CAD build for the part. Positions are in the model's coordinates, mm. Round coordinates to 2 decimals unless told otherwise and drop trailing zeros. Loops run counter-clockwise (first coordinate to the right, second up) from the corner with the lowest first, then second, coordinate; pieces in that order, holes last. Notation, with made-up numbers: M 39.25,51.5 L 77.25,51.5 A14 ccw 77.25,75.5 Z; hole C 47,10 d8. An arc over 180 degrees is marked long. Put each result on its own line as item: value. Start each with the question number.
from build123d import *

# Parameters (mm, degrees)
BOSS_EXTRUDE1_DEPTH = 6.35
BOSS_EXTRUDE1_DRAFT = -5
CUT_EXTRUDE3_DEPTH  = 15.892070037
CIRPATTERN3_COUNT   = 12
BOSS_EXTRUDE3_DEPTH = 6.35
BOSS_EXTRUDE3_DRAFT = -5
FILLET2_R           = 0.381
BOSS_EXTRUDE4_REACH = 16.734
SKETCH8_R           = 1.1811
SKETCH9_R           = 1.1811
CUT_EXTRUDE4_DEPTH  = 15.73364215
CIRPATTERN4_COUNT   = 4


with BuildPart() as part:
    # Sketch1 → Boss-Extrude1 (with draft: the straight prism first)
    with BuildSketch(Plane(origin=(0, 0, 0), x_dir=(1, 0, 0), z_dir=(0, 1, 0))):
        with BuildLine():
            Line((-6.35, -9.525), (6.35, -9.525))
            ThreePointArc((6.35, -9.525), (8.59506403, -8.59506403), (9.525, -6.35))
            Line((9.525, -6.35), (9.525, 6.35))
            ThreePointArc((9.525, 6.35), (8.59506403, 8.59506403), (6.35, 9.525))
            Line((6.35, 9.525), (-6.35, 9.525))
            ThreePointArc((-6.35, 9.525), (-8.59506403, 8.59506403), (-9.525, 6.35))
            Line((-9.525, 6.35), (-9.525, -6.35))
            ThreePointArc((-9.525, -6.35), (-8.59506403, -8.59506403), (-6.35, -9.525))
        make_face()
    extrude(amount=-BOSS_EXTRUDE1_DEPTH)
    # Boss-Extrude1: the draft: its side faces are tilted about the plane it starts from
    boss_extrude1_sides = [part.faces().sort_by_distance(p)[0] for p in [
        (-8.59506403, -3.175, 8.59506403),
        (0, -3.175, 9.525),
        (8.59506403, -3.175, 8.59506403),
        (9.525, -3.175, 0),
        (8.59506403, -3.175, -8.59506403),
        (0, -3.175, -9.525),
        (-8.59506403, -3.175, -8.59506403),
        (-9.525, -3.175, 0),
    ]]
    draft(boss_extrude1_sides, Plane(origin=(0, 0, 0), x_dir=(1, 0, 0), z_dir=(0, 1, 0)), BOSS_EXTRUDE1_DRAFT)

    # Sketch6 → Cut-Extrude3 (cut, through all)
    with BuildSketch(Plane(origin=(0, 0, 0), x_dir=(0.9659258262890681, 0, 0.25881904510252135), z_dir=(-0.25881904510252135, 0, 0.9659258262890681))):
        Polygon((0, -2.159), (-7.366, -9.525), (7.366, -9.525), align=None)
    cut_extrude3 = extrude(amount=-CUT_EXTRUDE3_DEPTH, mode=Mode.SUBTRACT)

    # CirPattern3: Cut-Extrude3 ×12 about axis
    cirpattern3_axis = Axis((0, 0, 0), (0, 1, 0))
    for i in range(1, CIRPATTERN3_COUNT):
        add(cut_extrude3.rotate(cirpattern3_axis, i * 360 / CIRPATTERN3_COUNT), mode=Mode.SUBTRACT)


with BuildPart() as boss_extrude3_tool:
    # Sketch7 → Boss-Extrude3 (with draft: the straight prism first)
    with BuildSketch(Plane(origin=(0, 0, 0), x_dir=(1, 0, 0), z_dir=(0, 1, 0))):
        with BuildLine():
            Line((-6.35, -9.525), (6.35, -9.525))
            ThreePointArc((6.35, -9.525), (8.59506403, -8.59506403), (9.525, -6.35))
            Line((9.525, -6.35), (9.525, 6.35))
            ThreePointArc((9.525, 6.35), (8.59506403, 8.59506403), (6.35, 9.525))
            Line((6.35, 9.525), (-6.35, 9.525))
            ThreePointArc((-6.35, 9.525), (-8.59506403, 8.59506403), (-9.525, 6.35))
            Line((-9.525, 6.35), (-9.525, -6.35))
            ThreePointArc((-9.525, -6.35), (-8.59506403, -8.59506403), (-6.35, -9.525))
        make_face()
        with BuildLine():
            Line((-6.35, -7.493), (6.35, -7.493))
            ThreePointArc((6.35, -7.493), (7.158223051, -7.158223051), (7.493, -6.35))
            Line((7.493, -6.35), (7.493, 6.35))
            ThreePointArc((7.493, 6.35), (7.158223051, 7.158223051), (6.35, 7.493))
            Line((6.35, 7.493), (-6.35, 7.493))
            ThreePointArc((-6.35, 7.493), (-7.158223051, 7.158223051), (-7.493, 6.35))
            Line((-7.493, 6.35), (-7.493, -6.35))
            ThreePointArc((-7.493, -6.35), (-7.158223051, -7.158223051), (-6.35, -7.493))
        make_face(mode=Mode.SUBTRACT)
    extrude(amount=-BOSS_EXTRUDE3_DEPTH)
    # Boss-Extrude3: the draft: its side faces are tilted about the plane it starts from
    boss_extrude3_sides = [boss_extrude3_tool.faces().sort_by_distance(p)[0] for p in [
        (0, -3.175, 9.525),
        (8.59506403, -3.175, 8.59506403),
        (9.525, -3.175, 0),
        (8.59506403, -3.175, -8.59506403),
        (0, -3.175, -9.525),
        (-8.59506403, -3.175, -8.59506403),
        (-9.525, -3.175, 0),
        (-8.59506403, -3.175, 8.59506403),
        (-7.158223051, -3.175, 7.158223051),
        (-7.493, -3.175, 0),
        (-7.158223051, -3.175, -7.158223051),
        (0, -3.175, -7.493),
        (7.158223051, -3.175, -7.158223051),
        (7.493, -3.175, 0),
        (7.158223051, -3.175, 7.158223051),
        (0, -3.175, 7.493),
    ]]
    draft(boss_extrude3_sides, Plane(origin=(0, 0, 0), x_dir=(1, 0, 0), z_dir=(0, 1, 0)), BOSS_EXTRUDE3_DRAFT)


with BuildPart() as part_1:
    add(part.part)

    # Boss-Extrude3: add boss_extrude3_tool
    add(boss_extrude3_tool.part)

    # Fillet2
    fillet2_edges = [part_1.edges().sort_by_distance(p)[0] for p in [
        (8.202228727, -6.35, -8.202228727),
        (8.202228727, -6.35, 8.202228727),
        (-8.202228727, -6.35, 8.202228727),
        (-8.202228727, -6.35, -8.202228727),
        (-8.969446987, -6.35, 0),
        (0, -6.35, -8.969446987),
        (0, -6.35, 8.969446987),
        (8.969446987, -6.35, 0),
        (-8.048553013, -6.35, 0),
        (-7.551058354, -6.35, 7.551058354),
        (0, -6.35, 8.048553013),
        (7.551058354, -6.35, 7.551058354),
        (8.048553013, -6.35, 0),
        (7.551058354, -6.35, -7.551058354),
        (0, -6.35, -8.048553013),
        (-7.551058354, -6.35, -7.551058354),
    ]]
    fillet(fillet2_edges, radius=FILLET2_R)

    # Sketch8 → Boss-Extrude4 (add, up to next)
    with BuildSketch(Plane(origin=(0, -5.969, 0), x_dir=(-1, 0, 0), z_dir=(0, -1, 0)), mode=Mode.PRIVATE) as boss_extrude4_sk1:
        with Locations((0, 7.493)):
            Circle(SKETCH8_R)
    boss_extrude4_tool1 = extrude(boss_extrude4_sk1.sketch, amount=-BOSS_EXTRUDE4_REACH, mode=Mode.PRIVATE) - part_1.part
    boss_extrude4 = boss_extrude4_tool1.solids().sort_by_distance((0, -5.969, -7.493))[0]
    add(boss_extrude4)

    # Sketch9 → Cut-Extrude4 (cut, through all)
    with BuildSketch(Plane.XZ.offset(5.969)):
        with Locations((0, -7.493)):
            Circle(SKETCH9_R)
    cut_extrude4 = extrude(amount=CUT_EXTRUDE4_DEPTH, mode=Mode.SUBTRACT)

    # CirPattern4: Boss-Extrude4, Cut-Extrude4 ×4 about axis
    cirpattern4_axis = Axis((0, 0, 0), (0, 1, 0))
    add([boss_extrude4.rotate(cirpattern4_axis, i * 360 / CIRPATTERN4_COUNT) for i in range(1, CIRPATTERN4_COUNT)])
    add([cut_extrude4.rotate(cirpattern4_axis, i * 360 / CIRPATTERN4_COUNT) for i in range(1, CIRPATTERN4_COUNT)], mode=Mode.SUBTRACT)


solid = part_1.part
(1) Cut at B-B on y = -5.5. List the corners of the cut face in (x, z), and give its area (3 significant figures).
(2) Drill centre lines: line 1 along X through (y, z) = (-3.5, -7); line 2 along Z through (x, y) = (-4.25, -2.75); line 3 along Z through (x, y) = (-7.5, -4). Where is each one in solid material? Low to high.
(3) Cut at A-A on z = 5. List the corners of the cut face in (x, y) (3 decimals), and give its area (3 significant figures).
(4) Cut at D-D on y = -1.5. List the corners of the cut face in (x, z), and give its area (3 significant figures).
(5) Cut at C-C on x = -5.25. List the corners of the cut face in (y, z) (3 decimals).
(6) Mould opens along Z. For faces 1 (the cylindrical face through (0.034, -4.45, -6.312)), 2 (the flat face through (-4.96, -2.83, -2.024)) say: +Z half, -Z half, draft (parallel to the pull), parting line (faces both ways), or undercut.
(7) Flat gauge pins, fed straight in: pin 1 Ø1.5 at (x, z) = (1, -2) entering from +Y; pin 2 Ø1 at (x, y) = (2, -4) entering from +Z; pin 3 Ø1.5 at (x, z) = (-4, -7) entering from -Y; pin 4 Ø1.2 at (x, z) = (0, 8) entering from -Y. Where does each tip first touch, or does it go through?
Taken from the geometry:
1. outline: M -9.04,-6.35 A2.69 ccw -6.35,-9.04 L 6.35,-9.04 A2.69 ccw 9.04,-6.35 L 9.04,6.35 A2.69 ccw 6.35,9.04 L -6.35,9.04 A2.69 ccw -9.04,6.35 Z; hole M -7.97,-6.35 A1.62 ccw -6.35,-7.97 L -1.08,-7.97 A1.18 cw long 1.08,-7.97 L 6.35,-7.97 A1.62 ccw 7.97,-6.35 L 7.97,-1.08 A1.18 cw long 7.97,1.08 L 7.97,6.35 A1.62 ccw 6.35,7.97 L 1.08,7.97 A1.18 cw long -1.08,7.97 L -6.35,7.97 A1.62 ccw -7.97,6.35 L -7.97,1.08 A1.18 cw long -7.97,-1.08 Z
1. area: 82.0 mm2
2. line 1: -9.14 to -7.65, -5.1 to -3.26, -1.07 to 1.07, 3.26 to 5.1, 7.65 to 9.14
2. line 2: -9.28 to -5.09, -3.41 to -1.75, -0.53 to 0.53, 1.75 to 3.41, 5.09 to 9.28
2. line 3: -8.93 to -7.3, -4.9 to -3.92, -1.18 to 1.18, 3.92 to 4.9, 7.3 to 8.93
3. outline: M -9.525,0 L -9,-6.002 A0.381 ccw -8.62,-6.35 L -8.398,-6.35 A0.381 ccw -8.018,-6.002 L -7.859,-4.18 L -5,-2.159 L -2.887,-3.653 L -1.34,-2.159 L 0,-3.453 L 1.34,-2.159 L 2.887,-3.653 L 5,-2.159 L 7.859,-4.18 L 8.018,-6.002 A0.381 ccw 8.398,-6.35 L 8.62,-6.35 A0.381 ccw 9,-6.002 L 9.525,0 Z
3. area: 64.0 mm2
4. outline: M -9.39,-6.35 A3.04 ccw -6.35,-9.39 L 6.35,-9.39 A3.04 ccw 9.39,-6.35 L 9.39,6.35 A3.04 ccw 6.35,9.39 L -6.35,9.39 A3.04 ccw -9.39,6.35 Z
4. area: 345 mm2
5. outline: M -6.35,-8.62 A0.381 ccw -6.002,-9 L 0,-9.525 L 0,9.525 L -6.002,9 A0.381 ccw -6.35,8.62 L -6.35,8.398 A0.381 ccw -6.002,8.018 L -3.992,7.842 L -2.159,5.25 L -3.728,3.031 L -2.159,1.407 L -3.518,0 L -2.159,-1.407 L -3.728,-3.031 L -2.159,-5.25 L -3.992,-7.842 L -6.002,-8.018 A0.381 ccw -6.35,-8.398 Z
6. face 1: undercut
6. face 2: undercut
7. pin 1: y = 0
7. pin 2: z = 9.22
7. pin 3: y = -4.44
7. pin 4: y = -5.97
